For this review, take the finished solid that the model builds, in its own axes (mm). A direction names the side the tool comes from. Round coordinates to 2 decimals unless told otherwise and drop trailing zeros. Write each loop counter-clockwise with the first axis right and the second up, starting at its lowest first coordinate (ties: lowest second). Pieces come first, ordered by that corner, then holes. Notation, with made-up numbers: M -4,-34.5 L 6,-34.5 A20 ccw 6,-2.5 Z; hole C 12,82 d7. An arc over 180 degrees is marked long. Answer in a Markdown table with one row per item.
```python
from build123d import *

# Parameters (mm, degrees)
SKETCH1_R           = 2.8575
BOSS_EXTRUDE1_DEPTH = 3.5052
CUT_EXTRUDE1_DEPTH  = 1.9558
SKETCH3_R           = 1.7145
BOSS_EXTRUDE2_DEPTH = 6.35


with BuildPart() as part:
    # Sketch1 → Boss-Extrude1 (new body)
    with BuildSketch(Plane(origin=(0, 0, 0), x_dir=(1, 0, 0), z_dir=(0, 1, 0))):
        Circle(SKETCH1_R)
    extrude(amount=BOSS_EXTRUDE1_DEPTH)

    # Sketch2 → Cut-Extrude1 (cut)
    with BuildSketch(Plane.XZ):
        Polygon((1.603951217, 0), (0.801975608, 1.3890625), (-0.801975608, 1.3890625), (-1.603951217, 0), (-0.801975608, -1.3890625), (0.801975608, -1.3890625), align=None)
    extrude(amount=-CUT_EXTRUDE1_DEPTH, mode=Mode.SUBTRACT)

    # Sketch3 → Boss-Extrude2 (add)
    with BuildSketch(Plane(origin=(0, 3.5052, 0), x_dir=(1, 0, 0), z_dir=(0, 1, 0))):
        Circle(SKETCH3_R)
    extrude(amount=BOSS_EXTRUDE2_DEPTH)


solid = part.part
```
Q1. Machinability: for faces 1 (the face through (-1.2, 1, 0.7)), 2 (the face through (0, 9.855, 0)), which of the approach directions +Z, -Z, +X, -X, +Y, -Y give a long, thin tool a straight path to every point of the face, cutting with its end or side? Answer none if there is none.
Found:
| item | result |
|---|---|
| face 1 | -Y |
| face 2 | +Z, -Z, +X, -X, +Y |
Q2. Take a section at A-A (x = 0). State the section outline as (y, z) points, then the cut area to 3 significant figures.
Found:
| item | result |
|---|---|
| outline | M 0,-2.86 L 3.51,-2.86 L 3.51,-1.71 L 9.86,-1.71 L 9.86,1.71 L 3.51,1.71 L 3.51,2.86 L 0,2.86 L 0,1.39 L 1.96,1.39 L 1.96,-1.39 L 0,-1.39 Z |
| area | 36.4 mm² |
Q3. Mouldability with a two-part tool opening along X and no side actions: class faces 3 (the face through (-0.372, 6.636, 1.674)), 4 (the face through (1.2, 1, 0.7)), 5 (the face through (0, 3.505, 2)) as +X half, -X half, draft (parallel to the pull), parting line (faces both ways), or undercut.
Found:
| item | result |
|---|---|
| face 3 | parting line |
| face 4 | undercut |
| face 5 | draft |
Q4. Take a section at C-C (y = 7.5). State the section outline as (x, z) points.
Found:
| item | result |
|---|---|
| outline | C 0,0 d3.43 |
Q5. For probe 1 along Y at (x, z) = (2.1, 0.25); probe 2 along Z at (x, y) = (0.1, 7.25), list the stretches that pass through material, from the lowest coordinate up.
Found:
| item | result |
|---|---|
| probe 1 | 0 to 3.51 |
| probe 2 | -1.71 to 1.71 |
Q6. Take a section at B-B (z = 0.25). State the section outline as (x, y) points, then the cut area to 3 significant figures.
Found:
| item | result |
|---|---|
| outline | M -2.85,0 L -1.46,0 L -1.46,1.96 L 1.46,1.96 L 1.46,0 L 2.85,0 L 2.85,3.51 L 1.7,3.51 L 1.7,9.86 L -1.7,9.86 L -1.7,3.51 L -2.85,3.51 Z |
| area | 35.8 mm² |
Q7. Take a section at D-D (x = 1.9). State the section outline as (y, z) points.
Found:
| item | result |
|---|---|
| outline | M 0,-2.13 L 3.51,-2.13 L 3.51,2.13 L 0,2.13 Z |
Q8. Insertion check: P1, Ø1.4, axis at x = -0.5, z = 0, coming from the -Y side; P2, Ø3, axis at x = -2, y = 4, coming from the +Z side; P3, Ø1.5, axis at x = 0, y = 5, coming from the -Z side. Each pin has a flat end and moves straight along its axis. Give the tip position at first contact, or say it passes through.
Found:
| item | result |
|---|---|
| P1 | y = 1.96 |
| P2 | z = 2.8 |
| P3 | z = -1.71 |
